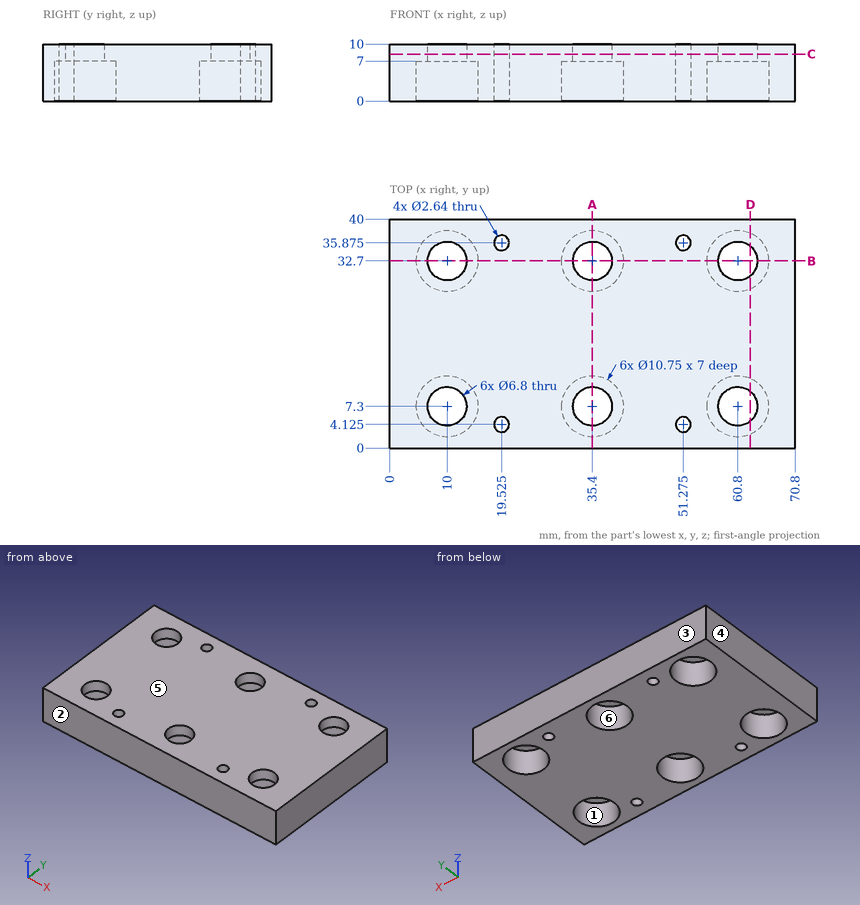
Job drawing, mm, ordinate dimensions from the low corner. One solid piece. A direction names the side the tool comes from. Round coordinates to 2 decimals unless told otherwise and drop trailing zeros. Loops run counter-clockwise (first coordinate to the right, second up) from the corner with the lowest first, then second, coordinate; pieces in that order, holes last. Notation, with made-up numbers: M -33.5,59 L 15.5,59 A17 ccw 15.5,64 Z; hole C -3,-27.75 d4. An arc over 180 degrees is marked long. Answer as CSV lines item,"result".
1. Cut at A-A on x = 35.4. Write the cut outline in (y, z) (3 decimals), then the cut area to 3 significant figures.
Resolved:
outline,"M 0,0 L 1.925,0 L 1.925,7 L 3.9,7 L 3.9,10 L 0,10 Z; M 10.7,7 L 12.675,7 L 12.675,0 L 27.325,0 L 27.325,7 L 29.3,7 L 29.3,10 L 10.7,10 Z; M 36.1,7 L 38.075,7 L 38.075,0 L 40,0 L 40,10 L 36.1,10 Z"
area,"209 mm²"
2. Wall check: probe 1 along Y at (x, z) = (60.8, 3.25) (3 decimals); probe 2 along Y at (x, z) = (11, 6.75); probe 3 along X at (y, z) = (10, 4.25). Give the ranges that are in metal, low to high. Write a range as [from, to].
Resolved:
probe 1,"y = [0, 1.925], [12.675, 27.325], [38.075, 40]"
probe 2,"y = [0, 2.02], [12.58, 27.42], [37.98, 40]"
probe 3,"x = [0, 5.35], [14.65, 30.75], [40.05, 56.15], [65.45, 70.8]"
3. Cut at B-B on y = 32.7. Write the cut outline in (x, z) (3 decimals), then the cut area to 3 significant figures.
Resolved:
outline,"M 0,0 L 4.625,0 L 4.625,7 L 6.6,7 L 6.6,10 L 0,10 Z; M 13.4,7 L 15.375,7 L 15.375,0 L 30.025,0 L 30.025,7 L 32,7 L 32,10 L 13.4,10 Z; M 38.8,7 L 40.775,7 L 40.775,0 L 55.425,0 L 55.425,7 L 57.4,7 L 57.4,10 L 38.8,10 Z; M 64.2,7 L 66.175,7 L 66.175,0 L 70.8,0 L 70.8,10 L 64.2,10 Z"
area,"421 mm²"
4. Two-plate mould, pull along Y, no slides. Class the marked faces 1, 2, 3 and 4: released by +Y, released by -Y, zero draft, split by the parting line, or undercut.
Resolved:
face 1,"undercut"
face 2,"released by -Y"
face 3,"released by +Y"
face 4,"zero draft"
5. Cut at D-D on x = 63. Write the cut outline in (y, z).
Resolved:
outline,"M 0,0 L 2.4,0 L 2.4,7 L 4.71,7 L 4.71,10 L 0,10 Z; M 9.89,7 L 12.2,7 L 12.2,0 L 27.8,0 L 27.8,7 L 30.11,7 L 30.11,10 L 9.89,10 Z; M 35.29,7 L 37.6,7 L 37.6,0 L 40,0 L 40,10 L 35.29,10 Z"
6. 3-axis set-ups, long thin cutter, end or side, ignore diameter. For the marked faces 5 and 6: which of +Z, -Z, +X, -X, +Y, -Y reach the whole face in a straight line?
Resolved:
face 5,"+Z, +X, -X, +Y, -Y"
face 6,"-Z"
7. Flat gauge pin, fed straight in: P1, Ø9, axis at x = 60.8, y = 32.7, coming from the -Z side. Where does the tip first touch, or does it go through?
Resolved:
P1,"stops at z = 7"
8. Cut at C-C on z = 8.25. Count the separate pieces of the cut face and the enclosed holes in it, then the cut area to 3 significant figures.
Resolved:
separate pieces,"1"
enclosed holes,"10"
area,"2,590 mm²"
